Check sheet for the modelled part. Datum: model origin and axes. Units: mm. Face numbers are marked on the shaded views. A direction names the side the tool comes from. Coordinates: 2 decimals unless noted, no trailing zeros. Loops run counter-clockwise (first coordinate to the right, second up) from the corner with the lowest first, then second, coordinate; pieces in that order, holes last. Notation, with made-up numbers: (85.25, 7) - (118.25, 7) arc R24 ccw to (118.25, 17) - close; hole circle Ø5 at (74.5, -13). An arc over 180 degrees is marked (long way). Use a Markdown table: item, result. Add a question column.
1) Thickness scan on line 1 (X direction, y = -9, z = -44); line 2 (Z direction, x = -24.5, y = -8.55); line 3 (Y direction, x = 51, z = -14.5). Record the ranges inside material, lowest first.
2) Sectioned sample at D-D, the plane z = -52. Enter the section's corners in (x, y), then the cut area to 3 significant figures.
3) Go/stop test with flat-tipped pins: P1, Ø11, axis at x = -27, z = -42, coming from the +Y side; P2, Ø1.5, axis at x = 7, y = -1.5, coming from the +Z side; P3, Ø4.5, axis at y = -1.5, z = -42, coming from the -X side. Record where each tip stops, or that it passes through.
4) Tool access check on the marked faces 1, 2 and 3. Record the directions out of +Z, -Z, +X, -X, +Y, -Y that give a thin tool (end or side, any length) a straight path to the whole face; none if there is none.
5) Sectioned sample at B-B, the plane y = 8. Enter the section's corners in (x, z), then the cut area to 3 significant figures.
6) Sectioned sample at A-A, the plane y = -8.5. State how many separate pieces and enclosed holes the cut face has, then the cut area to 3 significant figures.
7) Draft check along X on the marked faces 4, 5 and 6. Enter one of: pulls with the +X half, pulls with the -X half, needs draft (parallel to the pull), parting line crosses it, or undercut.
8) Sectioned sample at C-C, the plane y = 1.75. Enter the section's corners in (x, z), then the cut area to 3 significant figures.
Autodesk Inventor part; units mm, degrees
ref_plane "YZ Plane" through (0, 0, 0) normal (1, 0, 0) x (0, 1, 0)
ref_plane "XZ Plane" through (0, 0, 0) normal (0, 1, 0) x (-1, 0, 0)
ref_plane "XY Plane" through (0, 0, 0) normal (0, 0, 1) x (1, 0, 0)
sketch "Sketch1" plane through (0, 0, 0) normal (0, 1, 0) x (-1, 0, 0)
  circle A0 centre (0, 0) radius 60
  line L0 (14.7721, 2.6047) -> (41.3619, 7.2932)
  line L1 (14.7721, -2.6047) -> (41.3619, -7.2932)
  line L2 (0, 0) -> (115.9423, 0) construction
  line L3 (0, 0) -> (87.3255, -15.3978) construction
  line L4 (5.1303, 14.0954) -> (14.3648, 39.4671)
  line L5 (9.6418, 11.4907) -> (26.9971, 32.1739)
  line L6 (-9.6418, 11.4907) -> (-26.9971, 32.1739)
  line L7 (-5.1303, 14.0954) -> (-14.3648, 39.4671)
  line L8 (-14.7721, -2.6047) -> (-41.3619, -7.2932)
  line L9 (-14.7721, 2.6047) -> (-41.3619, 7.2932)
  line L10 (-5.1303, -14.0954) -> (-14.3648, -39.4671)
  line L11 (-9.6418, -11.4907) -> (-26.9971, -32.1739)
  line L12 (9.6418, -11.4907) -> (26.9971, -32.1739)
  line L13 (5.1303, -14.0954) -> (14.3648, -39.4671)
  arc A1 (41.3619, 7.2932) -> (26.9971, 32.1739) centre (0, 0) ccw
  arc A2 (26.9971, -32.1739) -> (41.3619, -7.2932) centre (0, 0) ccw
  arc A3 (-14.3648, -39.4671) -> (14.3648, -39.4671) centre (0, 0) ccw
  arc A4 (-41.3619, -7.2932) -> (-26.9971, -32.1739) centre (0, 0) ccw
  arc A5 (14.3648, 39.4671) -> (-14.3648, 39.4671) centre (0, 0) ccw
  arc A6 (-26.9971, 32.1739) -> (-41.3619, 7.2932) centre (0, 0) ccw
  circle A7 centre (0, 0) radius 42 construction
  circle A8 centre (0, 0) radius 15 construction
  arc A9 (9.6418, -11.4907) -> (14.7721, -2.6047) centre (0, 0) ccw
  arc A10 (-5.1303, -14.0954) -> (5.1303, -14.0954) centre (0, 0) ccw
  arc A11 (-14.7721, -2.6047) -> (-9.6418, -11.4907) centre (0, 0) ccw
  arc A12 (-9.6418, 11.4907) -> (-14.7721, 2.6047) centre (0, 0) ccw
  arc A13 (14.7721, 2.6047) -> (9.6418, 11.4907) centre (0, 0) ccw
  arc A14 (5.1303, 14.0954) -> (-5.1303, 14.0954) centre (0, 0) ccw
  dimension "d12" = 30
  dimension "d13" = 84
  dimension "d0" = 120
  dimension "d3" = 20
  dimension "d4" = 10
  dimension "d10" = 360
extrude "Extrusion1" add sketch "Sketch1" against normal blind 10
sketch "Sketch2" plane through (0, 0, 0) normal (0, 1, 0) x (1, 0, 0)
  circle A0 centre (-49, 0) radius 4
  line L0 (0, 0) -> (-95.2262, 0) construction
  line L1 (-49, 8.0829) -> (-42, 4.0415)
  line L2 (-42, 4.0415) -> (-42, -4.0415)
  line L3 (-42, -4.0415) -> (-49, -8.0829)
  line L4 (-49, -8.0829) -> (-56, -4.0415)
  line L5 (-56, -4.0415) -> (-56, 4.0415)
  line L6 (-56, 4.0415) -> (-49, 8.0829)
  line L7 (0, 0) -> (0, 100.6491) construction
  circle A1 centre (-24.5, -42.4352) radius 4
  line L8 (-31.5, -38.3938) -> (-24.5, -34.3523)
  line L9 (-24.5, -34.3523) -> (-17.5, -38.3938)
  line L10 (-17.5, -38.3938) -> (-17.5, -46.4767)
  line L11 (-17.5, -46.4767) -> (-24.5, -50.5181)
  line L12 (-24.5, -50.5181) -> (-31.5, -46.4767)
  line L13 (-31.5, -46.4767) -> (-31.5, -38.3938)
  circle A2 centre (24.5, -42.4352) radius 4
  line L14 (17.5, -46.4767) -> (17.5, -38.3938)
  line L15 (17.5, -38.3938) -> (24.5, -34.3523)
  line L16 (24.5, -34.3523) -> (31.5, -38.3938)
  line L17 (31.5, -38.3938) -> (31.5, -46.4767)
  line L18 (31.5, -46.4767) -> (24.5, -50.5181)
  line L19 (24.5, -50.5181) -> (17.5, -46.4767)
  circle A3 centre (49, 0) radius 4
  line L20 (49, -8.0829) -> (42, -4.0415)
  line L21 (42, -4.0415) -> (42, 4.0415)
  line L22 (42, 4.0415) -> (49, 8.0829)
  line L23 (49, 8.0829) -> (56, 4.0415)
  line L24 (56, 4.0415) -> (56, -4.0415)
  line L25 (56, -4.0415) -> (49, -8.0829)
  circle A4 centre (24.5, 42.4352) radius 4
  line L26 (31.5, 38.3938) -> (24.5, 34.3523)
  line L27 (24.5, 34.3523) -> (17.5, 38.3938)
  line L28 (17.5, 38.3938) -> (17.5, 46.4767)
  line L29 (17.5, 46.4767) -> (24.5, 50.5181)
  line L30 (24.5, 50.5181) -> (31.5, 46.4767)
  line L31 (31.5, 46.4767) -> (31.5, 38.3938)
  circle A5 centre (-24.5, 42.4352) radius 4
  line L32 (-17.5, 46.4767) -> (-17.5, 38.3938)
  line L33 (-17.5, 38.3938) -> (-24.5, 34.3523)
  line L34 (-24.5, 34.3523) -> (-31.5, 38.3938)
  line L35 (-31.5, 38.3938) -> (-31.5, 46.4767)
  line L36 (-31.5, 46.4767) -> (-24.5, 50.5181)
  line L37 (-24.5, 50.5181) -> (-17.5, 46.4767)
  dimension "d16" = 8
  dimension "d17" = 49
  dimension "d18" = 14
  dimension "d21" = 360
extrude "Extrusion2" cut sketch "Sketch2" against normal blind 4 contours A0 | L1 L2 L3 L4 L5 L6 | A1 | L8 L9 L10 L11 L12 L13 | A2 | L14 L15 L16 L17 L18 L19 | A3 | L20 L21 L22 L23 L24 L25 | A4 | L26 L27 L28 L29 L30 L31 | A5 | L32 L33 L34 L35 L36 L37
extrude "Extrusion3" cut sketch "Sketch2" against normal through all contours A0 | A1 | A2 | A3 | A4 | A5
sketch "Sketch3" plane through (0, -10, 0) normal (0, -1, 0) x (1, 0, 0)
  circle A0 centre (0, 0) radius 11
  dimension "d27" = 22
extrude "Extrusion4" add sketch "Sketch3" along normal blind 5 and the other way blind 20
sketch "Sketch4" plane through (0, -15, 0) normal (0, -1, 0) x (1, 0, 0)
  arc A0 (-1.5, 2) -> (1.5, 2) centre (0, 0) ccw
  line L0 (-1.5, 2) -> (1.5, 2)
  dimension "d30" = 5
  dimension "d31" = 2
extrude "Extrusion5" cut sketch "Sketch4" against normal blind 20
properties part number "Reaction_wheel_3DPrint"
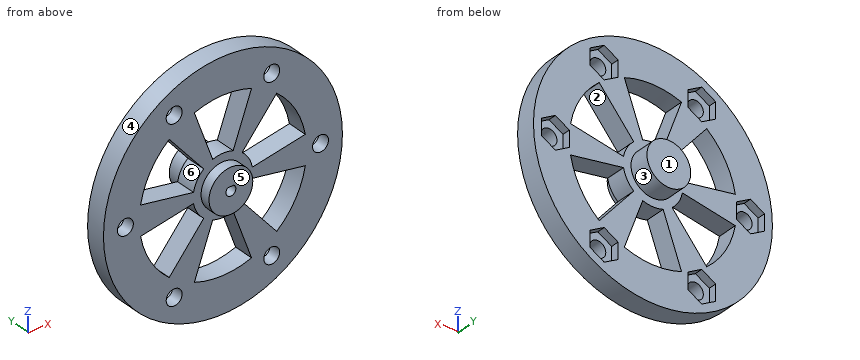
Solved:
| question | item | result |
|---|---|---|
| 1 | line 1 | x = -40.79 to -28.18, -20.82 to 20.82, 28.18 to 40.79 |
| 1 | line 2 | z = -54.77 to -46.44, -38.44 to -29.2, -4.32 to 4.32, 29.2 to 38.44, 46.44 to 54.77 |
| 1 | line 3 | y = -10 to 0 |
| 2 | outline | (-29.93, -10) - (29.93, -10) - (29.93, 0) - (-29.93, 0) - close |
| 2 | area | 599 mm2 |
| 3 | P1 | stops at y = 0 |
| 3 | P2 | stops at z = 59.67 |
| 3 | P3 | stops at x = -44.94 |
| 4 | face 1 | +Z, -Z, +X, -X, +Y |
| 4 | face 2 | +Y, -Y |
| 4 | face 3 | +Y |
| 5 | outline | circle Ø22 at (0, 0) |
| 5 | area | 380 mm2 |
| 6 | separate pieces | 1 |
| 6 | enclosed holes | 13 |
| 6 | area | 7,770 mm2 |
| 7 | face 4 | parting line crosses it |
| 7 | face 5 | needs draft |
| 7 | face 6 | undercut |
| 8 | outline | circle Ø22 at (0, 0); hole (-1.5, 2) arc R2.5 ccw (long way) to (1.5, 2) - close |
| 8 | area | 362 mm2 |
